from build123d import *

# Parameters (mm, degrees)
SKETCH_1_R      = 5
EXTRUDE_1_DEPTH = 9
SKETCH_5_R      = 5
EXTRUDE_5_DEPTH = 8
SKETCH_6_R      = 15
EXTRUDE_6_DEPTH = 4
CHAMFER_3_SIZE  = 1


with BuildPart() as part:
    # 草图1 → 凸台-拉伸1 (new body)
    with BuildSketch(Plane(origin=(0, 0, 0), x_dir=(1, 0, 0), z_dir=(0, 1, 0))):
        with Locations(Location((0, 0, 0), (0, 0, 270))):
            Circle(SKETCH_1_R)
        with BuildLine():
            Line((2.577287197, 1.63097845), (-2.485447743, 1.767780959))
            ThreePointArc((-2.485447743, 1.767780959), (-0.082385393, -3.048887116), (2.577287197, 1.63097845))
        make_face(mode=Mode.SUBTRACT)
    extrude(amount=EXTRUDE_1_DEPTH)

    # 草图5 → 凸台-拉伸5 (add)
    with BuildSketch(Plane(origin=(0, 9, 0), x_dir=(1, 0, 0), z_dir=(0, 1, 0))):
        with Locations(Location((0, 0, 0), (0, 0, 270))):
            Circle(SKETCH_5_R)
    extrude(amount=EXTRUDE_5_DEPTH)

    # 草图6 → 凸台-拉伸6 (add)
    with BuildSketch(Plane(origin=(0, 17, 0), x_dir=(1, 0, 0), z_dir=(0, 1, 0))):
        with Locations(Location((0, 0, 0), (0, 0, 270))):
            Circle(SKETCH_6_R)
    extrude(amount=EXTRUDE_6_DEPTH)

    # 倒角3
    chamfer_3_edges = [part.edges().sort_by_distance(p)[0] for p in [
        (0, 17, -5),
    ]]
    chamfer(chamfer_3_edges, length=CHAMFER_3_SIZE)


solid = part.part
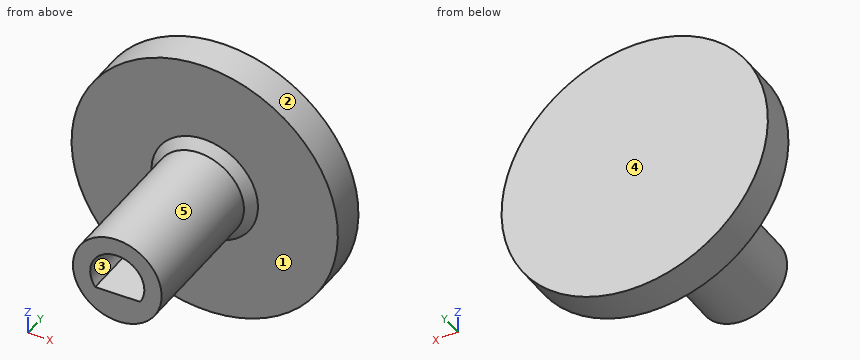
Verification items for the finished model (mm, model axes). Face numbers are marked on the shaded views. A direction names the side the tool comes from. Coordinates: 2 decimals unless noted, no trailing zeros. Order: outer loops, then holes, each group sorted by start corner. A loop starts at its lowest first (then second) coordinate and runs counter-clockwise, first axis right, second up. Notation, with made-up numbers: M 82.25,81 L 121.25,81 A15 cw 121.25,101 Z; hole C 17.5,-29 d11. An arc over 180 degrees is marked long. Write each question's results on one line, items separated by ' | '.
1) Scan lines: line 1 along X through (y, z) = (5.5, 0); line 2 along Y through (x, z) = (-13.25, -4.25); line 3 along X through (y, z) = (8.5, -1.5). Record each from-to range of solid material in increasing order. Write a range as [from, to].
Solved:
line 1: x = [-5, -3.05], [3.05, 5] | line 2: y = [17, 21] | line 3: x = [-4.77, -2.66], [2.66, 4.77]
2) Section check B-B on x = 0. Record the cut outline in (y, z), plus the area to 3 significant figures.
Solved:
outline: M 0,-5 L 16,-5 L 17,-6 L 17,-15 L 21,-15 L 21,15 L 17,15 L 17,6 L 16,5 L 0,5 L 0,3.05 L 9,3.05 L 9,-1.7 L 0,-1.7 Z | area: 248 mm²
3) Gauge pin test, flat ends, axial feed: pin 1 Ø1.4 at (x, z) = (-1, 0.5) entering from -Y; pin 2 Ø5 at (y, z) = (16.5, -4.5) entering from -X; pin 3 Ø10 at (y, z) = (10, -5.5) entering from -X; pin 4 Ø9 at (x, z) = (5, -7) entering from -Y. Record the tip position at first contact, or that the pin passes through.
Solved:
pin 1: stops at y = 9 | pin 2: stops at x = -14.86 | pin 3: stops at x = -4.97 | pin 4: stops at y = 0
4) Access from +Z, -Z, +X, -X, +Y, -Y to the whole of each face (thin tool, end or side, straight path). Record for the marked faces 1 and 2.
Solved:
face 1: -Y | face 2: +Y, -Y
5) Section check A-A on z = 0. Record the cut outline in (x, y), plus the area to 3 significant figures.
Solved:
outline: M -15,17 L -6,17 L -5,16 L -5,0 L -3.05,0 L -3.05,9 L 3.05,9 L 3.05,0 L 5,0 L 5,16 L 6,17 L 15,17 L 15,21 L -15,21 Z | area: 236 mm²
6) Section check C-C on y = 4. Record the cut outline in (x, z).
Solved:
outline: C 0,0 d10; hole M -2.49,-1.77 L 2.58,-1.63 A3.05 ccw long Z
7) Section check D-D on y = 12. Record the cut outline in (x, z).
Solved:
outline: C 0,0 d10
8) Release check for a two-part mould opening along Z. For the marked faces 3, 4 and 5 record: pulls with the +Z half, pulls with the -Z half, needs draft (parallel to the pull), parting line crosses it, or undercut.
Solved:
face 3: undercut | face 4: needs draft | face 5: parting line crosses it
